Check sheet for the modelled part. Datum: model origin and axes. Units: mm. Give positions to 0.01 mm unless a question says otherwise; leave off trailing zeros. Order: outer loops, then holes, each group sorted by start corner. A loop starts at its lowest first (then second) coordinate and runs counter-clockwise, first axis right, second up.
from build123d import *

# Parameters (mm, degrees)
SKETCH2_W           = 37.5
SKETCH2_H           = 206
BOSS_EXTRUDE2_DEPTH = 3
LPATTERN1_COUNT     = 3
LPATTERN1_PITCH     = 37.5


with BuildPart() as part:
    # Sketch2 → Boss-Extrude2 (new body)
    with BuildSketch(Plane(origin=(0, 0, 0), x_dir=(0, 0, -1), z_dir=(1, 0, 0))):
        Rectangle(SKETCH2_W, SKETCH2_H)
        Polygon((18.75, 118), (18.75, 103), (-18.75, 103), (-18.75, 118), (-12, 118), (-11, 108), (11, 108), (12, 118), align=None)
    boss_extrude2 = extrude(amount=BOSS_EXTRUDE2_DEPTH)

    # LPattern1: Boss-Extrude2 ×3
    with Locations(*[(0, 0, i * LPATTERN1_PITCH) for i in range(1, LPATTERN1_COUNT)]):
        add(boss_extrude2)


solid = part.part
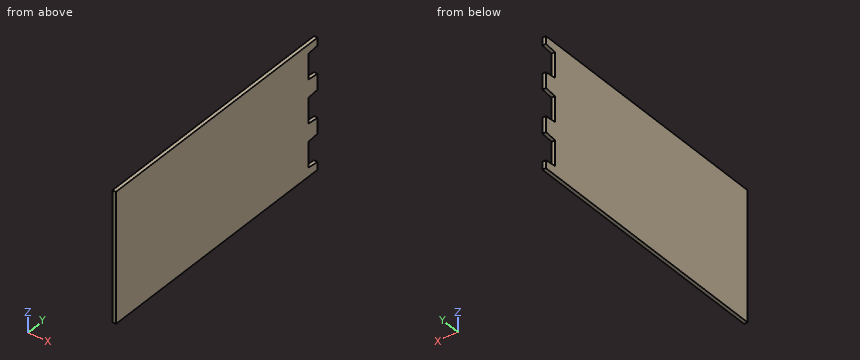
1) Material ranges on L1, parallel to Y at x = 0.55, z = 38, recorded low to high.
Recorded:
L1: y = -103 to 108
2) Section check A-A, the plane x = 2.2. Record the cut outline in (y, z), then the cut area to 3 significant figures.
Recorded:
outline: (-103, -18.75) - (118, -18.75) - (118, -12) - (108, -11) - (108, 11) - (118, 12) - (118, 25.5) - (108, 26.5) - (108, 48.5) - (118, 49.5) - (118, 63) - (108, 64) - (108, 86) - (118, 87) - (118, 93.75) - (-103, 93.75) - close
area: 24,200 mm2
3) Depth check by flat-ended pin: pin 1 Ø8 at (y, z) = (32.5, 71.5) entering from -X; pin 2 Ø1.5 at (x, z) = (1.5, 76.5) entering from +Y. Enter the tip coordinate at first touch or a pass-through.
Recorded:
pin 1: stops at x = 0
pin 2: stops at y = 108
4) Section check B-B, the plane z = -8. Record the cut outline in (x, y).
Recorded:
outline: (0, -103) - (3, -103) - (3, 108) - (0, 108) - close
